from build123d import *

# Parameters (mm, degrees)
F0_W     = 19.6
F0_H     = 19.6
F0_R     = 6
F1_DEPTH = 1
F2_W     = 19.6
F2_H     = 19.6
F2_W_2   = 17.6
F2_H_2   = 17.6
F3_DEPTH = 10.5


with BuildPart() as f1:
    # F0 (on Top) → F1 (new body)
    with BuildSketch(Plane.XY):
        Rectangle(F0_W, F0_H)
        Circle(F0_R, mode=Mode.SUBTRACT)
    extrude(amount=F1_DEPTH)

    # F2 (on face) → F3 (join)
    with BuildSketch(Plane(origin=(0, 0, 0), x_dir=(1, 0, 0), z_dir=(0, 0, -1))):
        Rectangle(F2_W, F2_H)
        Rectangle(F2_W_2, F2_H_2, mode=Mode.SUBTRACT)
    extrude(amount=F3_DEPTH)


solid = f1.part
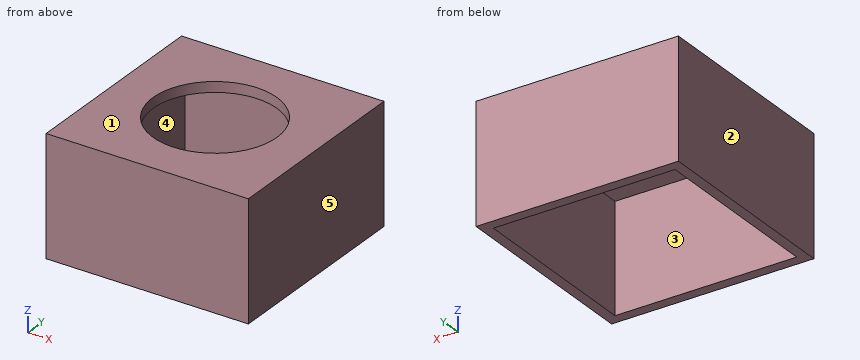
Geometry: final body of the model. Coordinates: model frame, mm. Face numbers are marked on the shaded views. A direction names the side the tool comes from. Give positions to 0.01 mm unless a question says otherwise; leave off trailing zeros. Order: outer loops, then holes, each group sorted by start corner. A loop starts at its lowest first (then second) coordinate and runs counter-clockwise, first axis right, second up. Notation, with made-up numbers: (38, 72) -> (56, 72) arc R35 cw to (56, 109) -> close; hole circle Ø3 at (57.25, -15.5). An arc over 180 degrees is marked (long way). Write each question's results on one line, items separated by ' | '.
1) Cut plane A-A (y = 0). Output: boundary loops of the cut face in (x, z), and give its area (3 significant figures).
Geometry says:
outline: (-9.8, -10.5) -> (-8.8, -10.5) -> (-8.8, 0) -> (-6, 0) -> (-6, 1) -> (-9.8, 1) -> close; (6, 0) -> (8.8, 0) -> (8.8, -10.5) -> (9.8, -10.5) -> (9.8, 1) -> (6, 1) -> close | area: 28.6 mm²
2) Set-up query: the marked faces 4 and 5. Return all of +Z, -Z, +X, -X, +Y, -Y with unobstructed straight access to the full face (end or side cutting, diameter ignored); none if empty.
Geometry says:
face 4: -Z | face 5: +Z, -Z, +X, +Y, -Y
3) Cut plane C-C (z = -8). Output: boundary loops of the cut face in (x, y).
Geometry says:
outline: (-9.8, -9.8) -> (9.8, -9.8) -> (9.8, 9.8) -> (-9.8, 9.8) -> close; hole (-8.8, -8.8) -> (8.8, -8.8) -> (8.8, 8.8) -> (-8.8, 8.8) -> close
4) First-contact query: pin 1 Ø5.5 at (x, y) = (4, 3.5) entering from -Z. Flat tip, straight axial feed; report the tip coordinate or a pass-through.
Geometry says:
pin 1: stops at z = 0
5) Draft query along X for the marked faces 1, 2 and 3. Return one class per face: released by +X, released by -X, zero draft, split by the parting line, or undercut.
Geometry says:
face 1: zero draft | face 2: released by -X | face 3: undercut
6) Line query: line 1 along Y through (x, z) = (0, 0.7); line 2 along Y through (x, z) = (-1.5, -3.75). Output: solid intervals per line, ascending.
Geometry says:
line 1: y = -9.8 to -6, 6 to 9.8 | line 2: y = -9.8 to -8.8, 8.8 to 9.8
7) Cut plane D-D (y = -7.25). Output: boundary loops of the cut face in (x, z).
Geometry says:
outline: (-9.8, -10.5) -> (-8.8, -10.5) -> (-8.8, 0) -> (8.8, 0) -> (8.8, -10.5) -> (9.8, -10.5) -> (9.8, 1) -> (-9.8, 1) -> close
